```python
from build123d import *


with BuildPart() as f1:
    # F0 (on Front) → F1 (revolve)
    with BuildSketch(Plane.XZ):
        with BuildLine():
            Line((-8.97, -53.276034), (0, -53.276034))
            Line((0, -53.276034), (0, 46.723966))
            Line((0, 46.723966), (0, 71.723966))
            Line((0, 71.723966), (-3.4, 71.723966))
            ThreePointArc((-3.4, 71.723966), (-4.814214, 71.138179), (-5.4, 69.723966))
            Line((-5.4, 69.723966), (-5.4, 48.223966))
            ThreePointArc((-5.4, 48.223966), (-5.83934, 47.163306), (-6.9, 46.723966))
            Line((-6.9, 46.723966), (-7.97, 46.723966))
            ThreePointArc((-7.97, 46.723966), (-8.677107, 46.431073), (-8.97, 45.723966))
            Line((-8.97, 45.723966), (-8.97, -53.276034))
        make_face()
        with BuildLine():
            Line((0, -73.276034), (0, -53.276034))
            Line((0, -53.276034), (-8.97, -53.276034))
            Line((-8.97, -53.276034), (-5.286714, -68.176575))
            add(Edge.make_bspline(
                [(0, -73.276034), (-3.358694, -72.929113), (-4.330067, -70.94463), (-5.286714, -68.176575)],
                knots=[0, 0, 0, 0, 7.345327, 7.345327, 7.345327, 7.345327], degree=3))
        make_face()
    revolve(axis=Axis((0, 0, -3.276034), (0, 0, 1)))


solid = f1.part
```
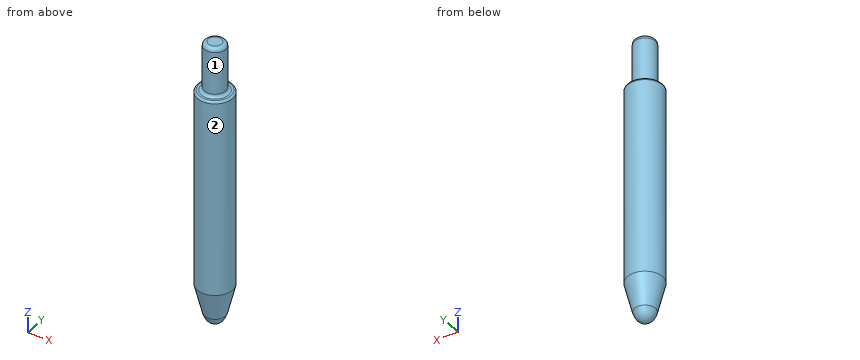
Input: part model. Units: mm. Frame: model coordinates. Face numbers are marked on the shaded views. A direction names the side the tool comes from. Give positions to 0.01 mm unless a question says otherwise; leave off trailing zeros. Loops run counter-clockwise (first coordinate to the right, second up) from the corner with the lowest first, then second, coordinate; pieces in that order, holes last. Notation, with made-up numbers: (29, 37.5) -> (61, 37.5) arc R31 ccw to (61, 61.5) -> close; hole circle Ø3 at (29.5, -10.5). An arc over 180 degrees is marked (long way). Use a Markdown table: item, result.
Q1. Access query for the marked faces 1 and 2. Directions: +Z, -Z, +X, -X, +Y, -Y. A direction counts if a zero-diameter tool reaches every point of the face in a straight line with its end or side. Return the directions, or none.
Entries:
| item | result |
|---|---|
| face 1 | +Z |
| face 2 | +Z, -Z |
Q2. Section query B-B, the plane z = 55. Return the cut outline in (x, y), plus the area to 3 significant figures.
Entries:
| item | result |
|---|---|
| outline | circle Ø10.8 at (0, 0) |
| area | 91.6 mm² |
Q3. First-contact query: P1, Ø1.5, axis at x = 2, z = -50.5, coming from the -Y side; P2, Ø6, axis at x = -3, z = -25.5, coming from the +Y side; P3, Ø1, axis at x = 2.5, z = 15, coming from the -Y side; P4, Ø6, axis at x = -3.5, y = -6.5, coming from the +Z side. Flat tips, straight axial feed; report the tip coordinate or a pass-through.
Entries:
| item | result |
|---|---|
| P1 | stops at y = -8.88 |
| P2 | stops at y = 8.97 |
| P3 | stops at y = -8.74 |
| P4 | stops at z = 71.47 |
Q4. Ray query, probe 1 along X at (y, z) = (5.75, -46); probe 2 along Y at (x, z) = (0.5, 55.5). Return the intervals inside material, ascending. Write a range as from..to.
Entries:
| item | result |
|---|---|
| probe 1 | x = -6.88..6.88 |
| probe 2 | y = -5.38..5.38 |
Q5. Section query A-A, the plane z = -16. Return the cut outline in (x, y), plus the area to 3 significant figures.
Entries:
| item | result |
|---|---|
| outline | circle Ø17.94 at (0, 0) |
| area | 253 mm² |
